Geometry: final body of the model. Coordinates: model frame, mm. A direction names the side the tool comes from. Give positions to 0.01 mm unless a question says otherwise; leave off trailing zeros.
```python
from build123d import *

# Parameters (mm, degrees)
F0_R            = 17.3565013667
F0_R_2          = 2.15265
F1_DEPTH        = 5.08
F3_DEPTH        = 5.08
F3_COPIES_COUNT = 35


# Not quite as in the source:
# - a pattern or mirror of a feature is missing from the dataset's text; its kind, count and spacing are read off the source's solid
# - a feature names something its author has since deleted; it is built from what else it names


with BuildPart() as f1:
    # F0 (on Top) → F1 (new body)
    with BuildSketch(Plane.XY):
        Circle(F0_R)
        with Locations((-9.6237072996, -5.55625)):
            Circle(F0_R_2, mode=Mode.SUBTRACT)
        with Locations((9.6237072996, -5.55625)):
            Circle(F0_R_2, mode=Mode.SUBTRACT)
        Polygon((6.4158048664, 0), (3.2079024332, -5.55625), (-3.2079024332, -5.55625), (-6.4158048664, 0), (-3.2079024332, 5.55625), (3.2079024332, 5.55625), align=None, mode=Mode.SUBTRACT)
        with Locations((0, 11.1125)):
            Circle(F0_R_2, mode=Mode.SUBTRACT)
    extrude(amount=F1_DEPTH)

    # F2 (on face) → F3 (cut, through all)
    with BuildSketch(Plane.XY.offset(5.08)):
        with BuildLine():
            Line((0.275157943, 15.3777549622), (1.0756124971, 17.3231405192))
            ThreePointArc((1.0756124971, 17.3231405192), (0, 17.3565013667), (-1.0756124971, 17.3231405192))
            Line((-1.0756124971, 17.3231405192), (-0.275157943, 15.3777549622))
            ThreePointArc((-0.275157943, 15.3777549622), (0, 15.1934323047), (0.275157943, 15.3777549622))
        make_face()
    f3 = extrude(amount=-F3_DEPTH, mode=Mode.SUBTRACT)

    # F3_copies: F3 ×35 about axis
    f3_copies_axis = Axis((0, 0, 0), (0, 0, 1))
    for i in range(1, F3_COPIES_COUNT):
        add(f3.rotate(f3_copies_axis, i * 360 / F3_COPIES_COUNT), mode=Mode.SUBTRACT)


solid = f1.part
```
Item 1: Line query: L1, parallel to Y at x = 0, z = 2.9; L2, parallel to X at y = 16.5, z = 2.85; L3, parallel to X at y = -4.5, z = 3.45. Output: solid intervals per line, ascending.
Found:
L1: y = -17.36 to -5.56, 5.56 to 8.96, 13.27 to 15.19
L2: x = -5.08 to -3.93, -2.19 to -0.74, 0.74 to 2.19, 3.93 to 5.08
L3: x = -16.08 to -11.5, -7.75 to -3.82, 3.82 to 7.75, 11.5 to 16.08
Item 2: Pin query (flat end, axial travel): pin 1 Ø2 at (x, z) = (-3.5, 2) entering from +Y. Return the tip coordinate at first contact, or that it passes through.
Found:
pin 1: stops at y = 16.85
Item 3: Section A-A, the plane z = 3.95. State how many separate pieces and enclosed holes the cut face has, plus the area to 3 significant figures.
Found:
separate pieces: 1
enclosed holes: 4
area: 700 mm2
Item 4: Pull-direction query (Y, two-part tool) for faces 6 (the face through (4.8, 2.8, 2.5)), 7 (the face through (6.37, 15.06, 2.58)), 8 (the face through (3.7, -15.93, 2.58)); classes: +Y half, -Y half, draft (parallel to the pull), parting line (faces both ways), or undercut.
Found:
face 6: undercut
face 7: +Y half
face 8: -Y half
Item 5: Reachability of faces 1 (the face through (-4.834, 2.739, 2.504)), 2 (the face through (-15.957, 6.828, 2.504)), 3 (the face through (-16.099, 2.857, 2.576)), 4 (the face through (0.67, 16.34, 2.58)), 5 (the face through (16.28, 1.53, 2.58)) from +Z, -Z, +X, -X, +Y, -Y: full face, straight path, thin tool, end or side. Return the list, or none.
Found:
face 1: +Z, -Z
face 2: +Z, -Z, -X, +Y
face 3: +Z, -Z, -X
face 4: +Z, -Z, +Y
face 5: +Z, -Z, +X
